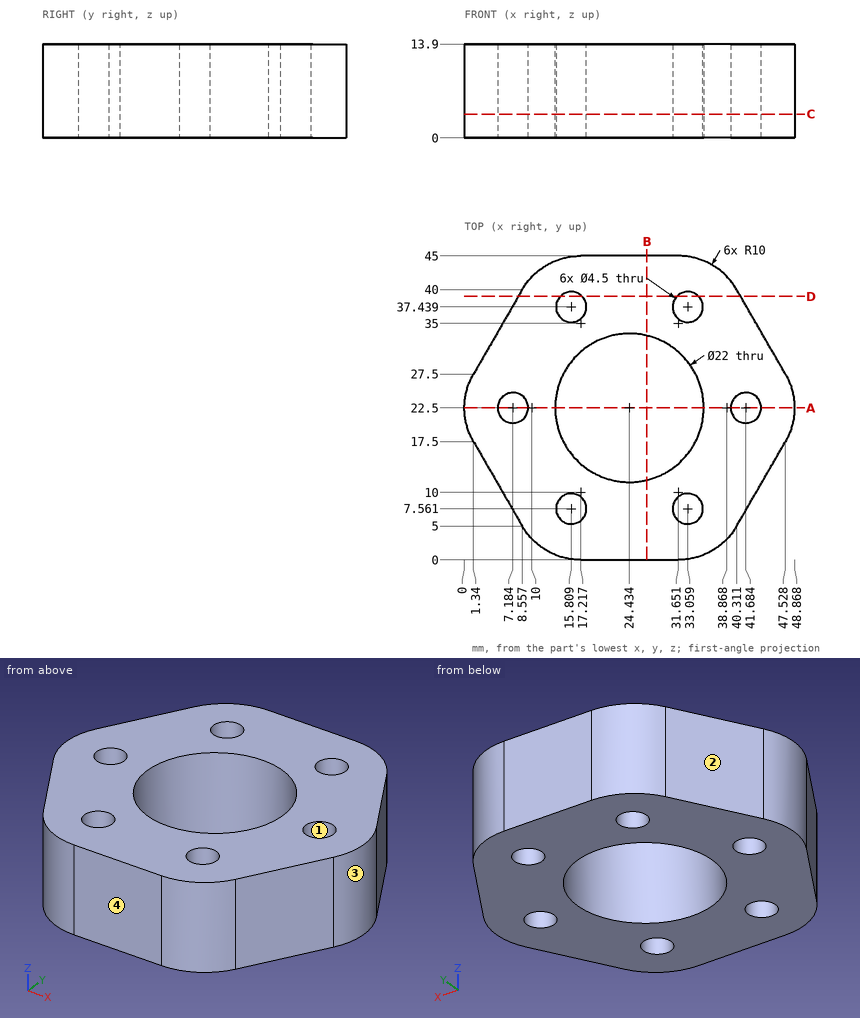
Geometry check sheet. Reference: drawing and pictorial views, mm from the part's lowest x, y, z. Give positions to 0.01 mm unless a question says otherwise; leave off trailing zeros. Order: outer loops, then holes, each group sorted by start corner. A loop starts at its lowest first (then second) coordinate and runs counter-clockwise, first axis right, second up. Notation, with made-up numbers: M 72.5,89 L 86.5,89 A30 ccw 86.5,121 Z; hole C 1.25,-11 d9. An arc over 180 degrees is marked long. Return JSON: item names as keys, results as strings. Group by question number.
1) Go/stop test with flat-tipped pins: pin 1 Ø2 at (y, z) = (10, 8.5) entering from -X; pin 2 Ø4 at (x, y) = (33.06, 37.44) entering from -Z; pin 3 Ø1 at (y, z) = (12.5, 11) entering from +X; pin 4 Ø5 at (x, z) = (40, 7.5) entering from -Y. Record where each tip stops, or that it passes through.
2) Section check B-B on x = 27. Record the cut outline in (y, z), and give its area (3 significant figures).
3) Section check A-A on y = 22.5. Record the cut outline in (x, z).
4) Mould release check, pull along Y, two halves, no side actions. Record for the marked faces 1, 2, 3 and 4: pulls with the +Y half, pulls with the -Y half, needs draft (parallel to the pull), parting line crosses it, or undercut.
5) Scan lines: line 1 (X direction, y = 37.5, z = 9.25) (1 decimal); line 2 (X direction, y = 23.5, z = 3.25); line 3 (Y direction, x = 19.5, z = 13). Record each from-to range of solid material in increasing order.
6) Section check D-D on y = 39. Record the cut outline in (x, z), and give its area (3 significant figures).
7) Section check C-C on z = 3.5. Record the cut outline in (x, y).
Answer block:
{
 "1": {"pin 1": "stops at x = 5.09", "pin 2": "passes through", "pin 3": "stops at x = 44.93", "pin 4": "stops at y = 1.89"},
 "2": {"outline": "M 0,0 L 11.8,0 L 11.8,13.9 L 0,13.9 Z; M 33.2,0 L 45,0 L 45,13.9 L 33.2,13.9 Z", "area": "328 mm^2"},
 "3": {"outline": "M 0,0 L 4.93,0 L 4.93,13.9 L 0,13.9 Z; M 9.43,0 L 13.43,0 L 13.43,13.9 L 9.43,13.9 Z; M 35.43,0 L 39.43,0 L 39.43,13.9 L 35.43,13.9 Z; M 43.93,0 L 48.87,0 L 48.87,13.9 L 43.93,13.9 Z"},
 "4": {"face 1": "undercut", "face 2": "pulls with the +Y half", "face 3": "parting line crosses it", "face 4": "pulls with the -Y half"},
 "5": {"line 1": "x = 7.1 to 13.6, 18.1 to 30.8, 35.3 to 41.8", "line 2": "x = 0.05 to 5.17, 9.2 to 13.48, 35.39 to 39.67, 43.7 to 48.82", "line 3": "y = 0 to 12.67, 32.33 to 45"},
 "6": {"outline": "M 7.98,0 L 14.19,0 L 14.19,13.9 L 7.98,13.9 Z; M 17.43,0 L 31.44,0 L 31.44,13.9 L 17.43,13.9 Z; M 34.68,0 L 40.89,0 L 40.89,13.9 L 34.68,13.9 Z", "area": "367 mm^2"},
 "7": {"outline": "M 1.34,17.5 L 8.56,5 A10 ccw 17.22,0 L 31.65,0 A10 ccw 40.31,5 L 47.53,17.5 A10 ccw 47.53,27.5 L 40.31,40 A10 ccw 31.65,45 L 17.22,45 A10 ccw 8.56,40 L 1.34,27.5 A10 ccw Z; hole C 7.18,22.5 d4.5; hole C 24.43,22.5 d22; hole C 15.81,7.56 d4.5; hole C 15.81,37.44 d4.5; hole C 33.06,7.56 d4.5; hole C 33.06,37.44 d4.5; hole C 41.68,22.5 d4.5"}
}
